Geometry: final body of the model. Coordinates: model frame, mm. Face numbers are marked on the shaded views. A direction names the side the tool comes from. Give positions to 0.01 mm unless a question says otherwise; leave off trailing zeros. Order: outer loops, then holes, each group sorted by start corner. A loop starts at its lowest first (then second) coordinate and runs counter-clockwise, first axis right, second up. Notation, with made-up numbers: (10.25, 35) - (60.25, 35) arc R26 cw to (60.25, 65) - close; hole circle Ø6 at (11, -18). An arc over 180 degrees is marked (long way). One line per question, with ' | ' between items. Start each with the question number.
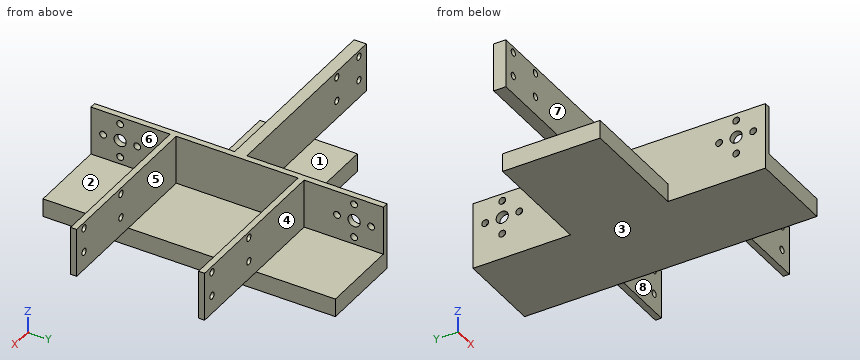
from build123d import *

# Parameters (mm, degrees)
SKETCH1_W           = 46
SKETCH1_H           = 40
SKETCH1_W_2         = 35
SKETCH1_H_2         = 120
BOSS_EXTRUDE2_DEPTH = 7.5
SKETCH2_W           = 46
SKETCH2_H           = 5
SKETCH2_W_2         = 32.5
SKETCH2_H_2         = 2.5
SKETCH2_W_3         = 35
BOSS_EXTRUDE3_DEPTH = 20
SKETCH3_R           = 1.4
CUT_EXTRUDE1_DEPTH  = 60
SKETCH4_R           = 1.4
CUT_EXTRUDE2_DEPTH  = 6
SKETCH6_R           = 1.4
SKETCH6_R_2         = 2.5
CUT_EXTRUDE3_DEPTH  = 2.5


with BuildPart() as part:
    # Sketch1 → Boss-Extrude2 (new body)
    with BuildSketch(Plane.XY):
        with Locations((-58, 0)):
            Rectangle(SKETCH1_W, SKETCH1_H)
        with Locations((-17.5, 0)):
            Rectangle(SKETCH1_W_2, SKETCH1_H_2)
    extrude(amount=BOSS_EXTRUDE2_DEPTH)

    # Sketch2 → Boss-Extrude3 (add)
    with BuildSketch(Plane.XY.offset(7.5)):
        with Locations((-58, 0)):
            Rectangle(SKETCH2_W, SKETCH2_H)
        Polygon((-32.5, 60), (-35, 60), (-35, 20), (-35, 2.5), (-35, -2.5), (-35, -20), (-35, -60), (-32.5, -60), (-32.5, -27.5), (-32.5, -25), (-32.5, 25), (-32.5, 27.5), align=None)
        with Locations((-16.25, 26.25)):
            Rectangle(SKETCH2_W_2, SKETCH2_H_2)
        with Locations((17.5, 26.25)):
            Rectangle(SKETCH2_W_3, SKETCH2_H_2)
        with Locations((17.5, -26.25)):
            Rectangle(SKETCH2_W_3, SKETCH2_H_2)
        with Locations((-16.25, -26.25)):
            Rectangle(SKETCH2_W_2, SKETCH2_H_2)
        with Locations((-98.5, 0)):
            Rectangle(SKETCH2_W_3, SKETCH2_H)
    extrude(amount=BOSS_EXTRUDE3_DEPTH)

    # Sketch3 → Cut-Extrude1 (cut)
    with BuildSketch(Plane.XZ.offset(27.5)):
        with Locations(Location((30, 25, 0), (0, 0, 180))):
            Circle(SKETCH3_R)
        with Locations(Location((30, 15, 0), (0, 0, 180))):
            Circle(SKETCH3_R)
        with Locations(Location((5, 25, 0), (0, 0, 180))):
            Circle(SKETCH3_R)
        with Locations(Location((5, 15, 0), (0, 0, 180))):
            Circle(SKETCH3_R)
    extrude(amount=-CUT_EXTRUDE1_DEPTH, mode=Mode.SUBTRACT)

    # Sketch4 → Cut-Extrude2 (cut)
    with BuildSketch(Plane.XZ.offset(2.5)):
        with Locations((-111, 25)):
            Circle(SKETCH4_R)
        with Locations((-96, 25)):
            Circle(SKETCH4_R)
        with Locations((-96, 15)):
            Circle(SKETCH4_R)
        with Locations((-111, 15)):
            Circle(SKETCH4_R)
    extrude(amount=-CUT_EXTRUDE2_DEPTH, mode=Mode.SUBTRACT)

    # Sketch6 → Cut-Extrude3 (cut)
    with BuildSketch(Plane(origin=(-32.5, 0, 0), x_dir=(0, 0, -1), z_dir=(1, 0, 0))):
        with Locations(Location((-24.5, -48, 0), (0, 0, 90))):
            Circle(SKETCH6_R)
        with Locations(Location((-17.5, -48, 0), (0, 0, 90))):
            Circle(SKETCH6_R_2)
        with Locations(Location((-17.5, -55, 0), (0, 0, 90))):
            Circle(SKETCH6_R)
        with Locations(Location((-17.5, -41, 0), (0, 0, 270))):
            Circle(SKETCH6_R)
        with Locations(Location((-10.5, -48, 0), (0, 0, 270))):
            Circle(SKETCH6_R)
        with Locations(Location((-10.5, 48, 0), (0, 0, 90))):
            Circle(SKETCH6_R)
        with Locations(Location((-17.5, 41, 0), (0, 0, 90))):
            Circle(SKETCH6_R)
        with Locations(Location((-17.5, 55, 0), (0, 0, 270))):
            Circle(SKETCH6_R)
        with Locations(Location((-17.5, 48, 0), (0, 0, 270))):
            Circle(SKETCH6_R_2)
        with Locations(Location((-24.5, 48, 0), (0, 0, 270))):
            Circle(SKETCH6_R)
    extrude(amount=-CUT_EXTRUDE3_DEPTH, mode=Mode.SUBTRACT)


solid = part.part
(1) Pull-direction query (Y, two-part tool) for the marked faces 6, 7 and 8; classes: +Y half, -Y half, draft (parallel to the pull), parting line (faces both ways), or undercut.
(2) Cut plane D-D, the plane z = 5.25. Return the cut outline in (x, y).
(3) Cut plane B-B, the plane y = 8. Return the cut outline in (x, z), plus the area to 4 significant figures.
(4) Cut plane C-C, the plane x = -8.5. Return the cut outline in (y, z), plus the area to 3 significant figures.
(5) Contact query for flat-ended pins moving along their axis: P1, Ø6, axis at y = -48, z = 17.5, coming from the -X side; P2, Ø6, axis at y = -37.5, z = 14.5, coming from the +X side; P3, Ø10, axis at x = -23, y = -50, coming from the +Z side. Output: stop coordinate, or through.
(6) Access query for the marked faces 1, 2, 3, 4 and 5. Directions: +Z, -Z, +X, -X, +Y, -Y. A direction counts if a zero-diameter tool reaches every point of the face in a straight line with its end or side. Return the directions, or none.
(7) Material intervals for line 1 along X through (y, z) = (25.7, 25); line 2 along Z through (x, y) = (-34, -48); line 3 along Z through (x, y) = (-96, 0.7), sorted ascending. Write a range as from..to.
(8) Cut plane A-A, the plane x = 12. Return the cut outline in (y, z), plus the area to 3 significant figures.
Results are:
1) face 6: draft | face 7: -Y half | face 8: undercut
2) outline: (-81, -20) - (-35, -20) - (-35, -60) - (0, -60) - (0, 60) - (-35, 60) - (-35, 20) - (-81, 20) - close
3) outline: (-81, 0) - (0, 0) - (0, 7.5) - (-32.5, 7.5) - (-32.5, 27.5) - (-35, 27.5) - (-35, 7.5) - (-81, 7.5) - close | area: 657.5 mm2
4) outline: (-60, 0) - (60, 0) - (60, 7.5) - (27.5, 7.5) - (27.5, 27.5) - (25, 27.5) - (25, 7.5) - (-25, 7.5) - (-25, 27.5) - (-27.5, 27.5) - (-27.5, 7.5) - (-60, 7.5) - close | area: 1,000 mm2
5) P1: x = -35 | P2: x = -32.5 | P3: z = 7.5
6) face 1: +Z, -X, +Y | face 2: +Z, +X, -Y | face 3: -Z, +X, -X, +Y, -Y | face 4: +Z, +X, +Y | face 5: +Z, +X
7) line 1: -35..3.6, 6.4..28.6, 31.4..35 | line 2: 0..9.1, 11.9..15, 20..23.1, 25.9..27.5 | line 3: 7.5..13.6, 16.4..23.6, 26.4..27.5
8) outline: (-27.5, 7.5) - (-25, 7.5) - (-25, 27.5) - (-27.5, 27.5) - close; (25, 7.5) - (27.5, 7.5) - (27.5, 27.5) - (25, 27.5) - close | area: 100 mm2
